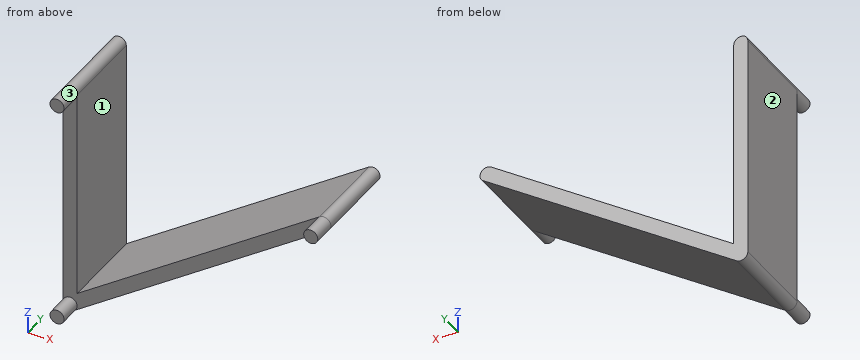
```python
from build123d import *

# Parameters (mm, degrees)
BOSS_EXTRUDE1_DEPTH = 38.1
BOSS_EXTRUDE2_START = 10.16
SKETCH2_R           = 3.175
BOSS_EXTRUDE2_DEPTH = 10.16


with BuildPart() as part:
    # Sketch1 → Boss-Extrude1 (new body)
    with BuildSketch(Plane(origin=(0, 0, 0), x_dir=(1, 0, 0), z_dir=(0, 1, 0))):
        with BuildLine():
            Line((-3.175, 0), (-3.175, 101.6))
            ThreePointArc((-3.175, 101.6), (-1.463672289, 104.417496838), (1.825496649, 104.197727273))
            Line((1.825496649, 104.197727273), (116.125496649, 23.875874704))
            ThreePointArc((116.125496649, 23.875874704), (116.897727273, 19.452650782), (112.474503351, 18.680420159))
            Line((112.474503351, 18.680420159), (3.175, 95.488281873))
            Line((3.175, 95.488281873), (3.175, 0))
            ThreePointArc((3.175, 0), (0, -3.175), (-3.175, 0))
        make_face()
    extrude(amount=BOSS_EXTRUDE1_DEPTH)

    # Sketch2 → Boss-Extrude2 (add)
    with BuildSketch(Plane(origin=(0, 0, 0), x_dir=(-1, 0, 0), z_dir=(0, -1, 0)).offset(BOSS_EXTRUDE2_START)):
        with Locations(Location((0, 0, 0), (0, 0, 90))):
            Circle(SKETCH2_R)
        with Locations(Location((0, 101.6, 0), (0, 0, 90))):
            Circle(SKETCH2_R)
        with Locations(Location((-114.3, 21.278147432, 0), (0, 0, 90))):
            Circle(SKETCH2_R)
    extrude(amount=-BOSS_EXTRUDE2_DEPTH)


solid = part.part
```
Verification items for the finished model (mm, model axes). Face numbers are marked on the shaded views. A direction names the side the tool comes from. Coordinates: 2 decimals unless noted, no trailing zeros. Loops run counter-clockwise (first coordinate to the right, second up) from the corner with the lowest first, then second, coordinate; pieces in that order, holes last. Notation, with made-up numbers: (-30.5, -33.75) - (23.5, -33.75) arc R20 cw to (23.5, -0.75) - close; hole circle Ø2 at (-35.5, 88.25). An arc over 180 degrees is marked (long way). Return JSON: item names as keys, results as strings.
1. Go/stop test with flat-tipped pins: pin 1 (10 mm diameter, centred on x = 57.5, y = 11.5, fed in from +Z); pin 2 (12 mm diameter, centred on x = 26, z = -78.5, fed in from -Y); pin 3 (10 mm diameter, centred on y = 29, z = -91, fed in from +X). Record where each tip stops, or that it passes through.
Established:
{"pin 1": "stops at z = -53.8", "pin 2": "stops at y = 0", "pin 3": "stops at x = 27.72"}
2. Section check C-C, the plane x = 0. Record the boundary of the cut face in (y, z) (3 decimals), then the cut area to 3 significant figures.
Established:
{"outline": "(-10.16, -104.775) - (38.1, -104.775) - (38.1, 3.175) - (-10.16, 3.175) - (-10.16, -3.175) - (0, -3.175) - (0, -98.425) - (-10.16, -98.425) - close", "area": "4,240 mm2"}
3. Tool access check on the marked faces 1, 2 and 3. Record the directions out of +Z, -Z, +X, -X, +Y, -Y that give a thin tool (end or side, any length) a straight path to the whole face; none if there is none.
Established:
{"face 1": "+Z, +Y, -Y", "face 2": "+Z, -Z, -X, +Y, -Y", "face 3": "-Y"}
4. Section check D-D, the plane x = 114.3. Record the boundary of the cut face in (y, z), then the cut area to 3 significant figures.
Established:
{"outline": "(-10.16, -24.45) - (0, -24.45) - (0, -25.16) - (38.1, -25.16) - (38.1, -18.1) - (-10.16, -18.1) - close", "area": "333 mm2"}
5. Thickness scan on L1, parallel to Y at x = 38.5, z = -74; L2, parallel to X at y = 21.5, z = -36 (3 decimals); L3, parallel to X at y = 32, z = -33 (3 decimals). Record the ranges inside material, lowest first.
Established:
{"L1": "y = 0 to 38.1", "L2": "x = -3.175 to 3.175, 87.828 to 98.873", "L3": "x = -3.175 to 3.175, 92.097 to 103.142"}
6. Section check B-B, the plane z = -64.5. Record the boundary of the cut face in (x, y) (3 decimals), then the cut area to 3 significant figures.
Established:
{"outline": "(-3.175, 0) - (3.175, 0) - (3.175, 38.1) - (-3.175, 38.1) - close; (47.272, 0) - (58.316, 0) - (58.316, 38.1) - (47.272, 38.1) - close", "area": "663 mm2"}
